```python
from build123d import *

# Parameters (mm, degrees)
F0_R     = 11.65
F1_DEPTH = 4
F2_R     = 1.99999
F3_R     = 3.25
F4_DEPTH = 25


# Not quite as in the source:
# - a fillet or chamfer is up to 0.001 mm smaller than in the source, because OpenCascade refuses the exact size


with BuildPart() as f1:
    # F0 (on Top) → F1 (new body)
    with BuildSketch(Plane.XY):
        Circle(F0_R)
    extrude(amount=F1_DEPTH)

    # F2 (radius 2 in the source; OpenCascade refuses exactly that, so slightly less here)
    f2_edges = [f1.edges().sort_by_distance(p)[0] for p in [
        (-11.65, 0, 4),
        (-11.65, 0, 0),
    ]]
    fillet(f2_edges, radius=F2_R)

    # F3 (on face) → F4 (cut)
    with BuildSketch(Plane.XY.offset(4)):
        Circle(F3_R)
    extrude(amount=-F4_DEPTH, mode=Mode.SUBTRACT)


solid = f1.part
```
Check sheet for the modelled part. Datum: model origin and axes. Units: mm. Give positions to 0.01 mm unless a question says otherwise; leave off trailing zeros. Loops run counter-clockwise (first coordinate to the right, second up) from the corner with the lowest first, then second, coordinate; pieces in that order, holes last. Notation, with made-up numbers: M 34,67 L 58,67 A26 cw 58,87 Z; hole C -36.5,-9 d9. An arc over 180 degrees is marked long. Answer as CSV lines item,"result".
Item 1: Sectioned sample at C-C, the plane z = 1.1. Enter the section's corners in (x, y).
Reply:
outline,"C 0,0 d22.87; hole C 0,0 d6.5"
Item 2: Draft check along Y on faces 1 (the face through (-2.579, -1.978, 2.028)), 2 (the face through (0, -4, 0)). Enter one of: pulls with the +Y half, pulls with the -Y half, needs draft (parallel to the pull), parting line crosses it, or undercut.
Reply:
face 1,"undercut"
face 2,"needs draft"
Item 3: Sectioned sample at D-D, the plane z = 3.65. Enter the section's corners in (x, y).
Reply:
outline,"C 0,0 d21.56; hole C 0,0 d6.5"
Item 4: Scan lines: L1, parallel to Y at x = 0, z = 2.25; L2, parallel to X at y = -1.5, z = 0.4; L3, parallel to Y at x = 0, z = 3.15. Record each from-to range of solid material in increasing order.
Reply:
L1,"-11.63 to -3.25, 3.25 to 11.63"
L2,"-10.75 to -2.88, 2.88 to 10.75"
L3,"-11.29 to -3.25, 3.25 to 11.29"
